from build123d import *

# Parameters (mm, degrees)
SKETCH_2_W          = 42
SKETCH_2_H          = 50
SKETCH_2_R          = 1.5
SKETCH_2_R_2        = 10
EXTRUDE_5_DEPTH     = 2
SKETCH_4_W          = 42
SKETCH_4_H          = 42
EXTRUDE_6_DEPTH     = 25
SKETCH_4_3_W        = 42
SKETCH_4_3_H        = 42
CUT_EXTRUDE_1_DEPTH = 23


with BuildPart() as part:
    # Sketch 2 → Extrude 5 (new body)
    with BuildSketch(Plane(origin=(0, 0, 0), x_dir=(0, 0, -1), z_dir=(1, 0, 0))):
        Rectangle(SKETCH_2_W, SKETCH_2_H)
        with Locations((15.5, 15.5)):
            Circle(SKETCH_2_R, mode=Mode.SUBTRACT)
        with Locations(Location((15.5, -15.5, 0), (0, 0, 180))):
            Circle(SKETCH_2_R, mode=Mode.SUBTRACT)
        with Locations((-15.5, -15.5)):
            Circle(SKETCH_2_R, mode=Mode.SUBTRACT)
        with Locations(Location((-15.5, 15.5, 0), (0, 0, 180))):
            Circle(SKETCH_2_R, mode=Mode.SUBTRACT)
        Circle(SKETCH_2_R_2, mode=Mode.SUBTRACT)
    extrude(amount=EXTRUDE_5_DEPTH)

    # Sketch 4 → Extrude 6 (add)
    with BuildSketch(Plane(origin=(0, 0, 0), x_dir=(1, 0, 0), z_dir=(0, 1, 0))):
        with Locations((-21, 0)):
            Rectangle(SKETCH_4_W, SKETCH_4_H)
        with BuildLine():
            Line((-37, 17.5), (-5, 17.5))
            ThreePointArc((-5, 17.5), (-3, 15.5), (-5, 13.5))
            Line((-5, 13.5), (-37, 13.5))
            ThreePointArc((-37, 13.5), (-39, 15.5), (-37, 17.5))
        make_face(mode=Mode.SUBTRACT)
        with BuildLine():
            Line((-37, -17.5), (-5, -17.5))
            ThreePointArc((-5, -17.5), (-3, -15.5), (-5, -13.5))
            Line((-5, -13.5), (-37, -13.5))
            ThreePointArc((-37, -13.5), (-39, -15.5), (-37, -17.5))
        make_face(mode=Mode.SUBTRACT)
    extrude(amount=EXTRUDE_6_DEPTH)

    # Sketch 4_3 → Cut-Extrude 1 (cut)
    with BuildSketch(Plane(origin=(0, 0, 0), x_dir=(1, 0, 0), z_dir=(0, 1, 0))):
        with Locations((-21, 0)):
            Rectangle(SKETCH_4_3_W, SKETCH_4_3_H)
        with BuildLine():
            Line((-37, 17.5), (-5, 17.5))
            ThreePointArc((-5, 17.5), (-3, 15.5), (-5, 13.5))
            Line((-5, 13.5), (-37, 13.5))
            ThreePointArc((-37, 13.5), (-39, 15.5), (-37, 17.5))
        make_face(mode=Mode.SUBTRACT)
        with BuildLine():
            Line((-37, -17.5), (-5, -17.5))
            ThreePointArc((-5, -17.5), (-3, -15.5), (-5, -13.5))
            Line((-5, -13.5), (-37, -13.5))
            ThreePointArc((-37, -13.5), (-39, -15.5), (-37, -17.5))
        make_face(mode=Mode.SUBTRACT)
    extrude(amount=CUT_EXTRUDE_1_DEPTH, mode=Mode.SUBTRACT)


solid = part.part
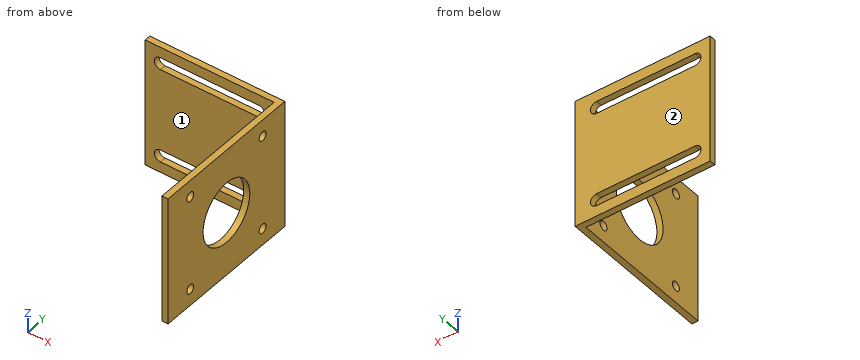
Can you work these out from the model? Positions are in its coordinate system, mm. Face numbers are marked on the shaded views. A direction names the side the tool comes from. Round coordinates to 2 decimals unless told otherwise and drop trailing zeros. Write each loop counter-clockwise with the first axis right and the second up, starting at its lowest first coordinate (ties: lowest second). Pieces come first, ordered by that corner, then holes. Notation, with made-up numbers: (86.25, -37) -> (114.25, -37) arc R24 ccw to (114.25, -27) -> close; hole circle Ø2 at (14.25, -24.5). An arc over 180 degrees is marked (long way). Use one line per item in the form item = value. Start each with the question number.
Q1. Imagine slicing it at B-B (x = -14). Please give me the cut outline in (y, z), then the cut area to 3 significant figures.
Q2. I'm going to push flat-ended pins straight in: P1, Ø1, axis at x = -4, z = 14, coming from the +Y side; P2, Ø8, axis at y = -11, z = 1.5, coming from the -X side; P3, Ø1.5, axis at x = -37, z = -6.5, coming from the -Y side. Where does each tip first touch, or does it pass through?
Q3. Imagine slicing it at D-D (z = 0). Please give me the cut outline in (x, y).
Q4. Which directions (+Z, -Z, +X, -X, +Y, -Y) give clear straight access to the entire face, cutting with the end or side of a thin tool? Please do the marked faces 1 and 2.
Q5. Imagine slicing it at A-A (y = 0). Please give me the cut outline in (x, z), then the cut area to 3 significant figures.
Q6. Imagine slicing it at C-C (z = 15.5). Please give me the cut outline in (x, y).
Q7. If I drill on probe 1 along Y at (x, z) = (1.35, 15.5); probe 2 along Y at (x, z) = (1.05, 0); probe 3 along X at (y, z) = (17.5, -2), over which ranges is the centre line in solid material (lowest first)? Write a range as [from, to].
Worked out:
q1.outline = (23, -21) -> (25, -21) -> (25, -17.5) -> (23, -17.5) -> close; (23, -13.5) -> (25, -13.5) -> (25, 13.5) -> (23, 13.5) -> close; (23, 17.5) -> (25, 17.5) -> (25, 21) -> (23, 21) -> close
q1.area = 68.0 mm^2
q2.P1 = 25
q2.P2 = 0
q2.P3 = 23
q3.outline = (-42, 23) -> (0, 23) -> (0, 10) -> (2, 10) -> (2, 25) -> (-42, 25) -> close; (0, -25) -> (2, -25) -> (2, -10) -> (0, -10) -> close
q4.face_1 = +Z, -Z, -X, -Y
q4.face_2 = +Z, -Z, +X, -X, +Y
q5.outline = (0, -21) -> (2, -21) -> (2, -10) -> (0, -10) -> close; (0, 10) -> (2, 10) -> (2, 21) -> (0, 21) -> close
q5.area = 44.0 mm^2
q6.outline = (-42, 23) -> (-39, 23) -> (-39, 25) -> (-42, 25) -> close; (-3, 23) -> (0, 23) -> (0, 17) -> (2, 17) -> (2, 25) -> (-3, 25) -> close; (0, -25) -> (2, -25) -> (2, -17) -> (0, -17) -> close; (0, -14) -> (2, -14) -> (2, 14) -> (0, 14) -> close
q7.probe_1 = [-25, -17], [-14, 14], [17, 25]
q7.probe_2 = [-25, -10], [10, 25]
q7.probe_3 = [0, 2]
